from build123d import *

# Parameters (mm, degrees)
SZKIC1_W                                            = 40
SZKIC1_H                                            = 20
POG_BIENIE_WALCOWE_POD_M8_WKR_T_Z_BEM_W_D           = 9
POG_BIENIE_WALCOWE_POD_M8_WKR_T_Z_BEM_W_CBORE_D     = 15
POG_BIENIE_WALCOWE_POD_M8_WKR_T_Z_BEM_W_CBORE_DEPTH = 8.6


with BuildPart() as part:
    # Szkic1 → Obrót1 (revolve)
    with BuildSketch(Plane.XY):
        with Locations((-130, -1.468948521)):
            Rectangle(SZKIC1_W, SZKIC1_H)
    revolve(axis=Axis((0, 8.531051479, 0), (0, -1, 0)))

    # Pogłębienie walcowe pod M8 Wkręt z łbem walcowym z gniazdem sześciokątnym1 (through all)
    with Locations(Plane(origin=(2.665933908, 8.531051479, 0), x_dir=(1, 0, 0), z_dir=(0, 1, 0))):
        with Locations((-139.982449122, 0), (-71.324191515, 118.919590535), (65.9923237, 118.919590535), (134.650581307, 0), (65.9923237, -118.919590535), (-71.324191515, -118.919590535)):
            CounterBoreHole(POG_BIENIE_WALCOWE_POD_M8_WKR_T_Z_BEM_W_D / 2, POG_BIENIE_WALCOWE_POD_M8_WKR_T_Z_BEM_W_CBORE_D / 2, POG_BIENIE_WALCOWE_POD_M8_WKR_T_Z_BEM_W_CBORE_DEPTH)


solid = part.part
Could you check a few things on this model? Use its own coordinates, in mm. A direction names the side the tool comes from. Give positions to 0.01 mm unless a question says otherwise; leave off trailing zeros. Order: outer loops, then holes, each group sorted by start corner. A loop starts at its lowest first (then second) coordinate and runs counter-clockwise, first axis right, second up. Notation, with made-up numbers: (1.5, 3) - (32.5, 3) arc R15 ccw to (32.5, 9) - close; hole circle Ø9 at (14, 38). An arc over 180 degrees is marked (long way). Return JSON: item names as keys, results as strings. Group by question number.
Q1. Suppose I cut it at C-C, the plane y = 3.5. Please give me the cut outline in (x, z).
Q2. Please list where these lines run through material, in increasing order: line 1 along X through (y, z) = (-1.25, -117.5); line 2 along X through (y, z) = (7, 124.5); line 3 along Z through (x, y) = (-71.5, 6.75). Write a range as [from, to].
Q3. Will these pins go through, and if not, where does the flat tip stop? pin 1 Ø8 at (y, z) = (2.5, 25) entering from -X; pin 2 Ø4.5 at (x, z) = (-70, -121.5) entering from +Y; pin 3 Ø1 at (y, z) = (-3, -53) entering from +X.
Q4. Thinking about a two-plate mould opening in Z: for faces 3 (the face through (66.58, -5.85, 122.91)), 4 (the face through (-65, -0.069, 122)), 5 (the face through (67, 8.531, 88)), 6 (the face through (19.527, -1.329, -148.724)), which applies, pulls with the +Z half, pulls with the -Z half, needs draft (parallel to the pull), parting line crosses it, or undercut?
Q5. Suppose I cut it at B-B, the plane z = 0. Please give me the cut outline in (x, y), and give its area (3 significant figures).
Q6. Which directions (+Z, -Z, +X, -X, +Y, -Y) give clear straight access to the entire face, cutting with the end or side of a thin tool? Please do faces 1 (the face through (141, -0.069, 3)), 2 (the face through (133.16, -5.85, 1.72)).
Q7. Suppose I cut it at A-A, the plane x = 0. Please give me the cut outline in (y, z).
Q8. Suppose I cut it at D-D, the plane z = 101. Please give me the cut outline in (x, y), and give its area (3 significant figures).
Resolved:
{
 "1": {"outline": "circle Ø300 at (0, 0); hole circle Ø15 at (-137.32, 0); hole circle Ø220 at (0, 0); hole circle Ø15 at (-68.66, -118.92); hole circle Ø15 at (-68.66, 118.92); hole circle Ø15 at (68.66, -118.92); hole circle Ø15 at (68.66, 118.92); hole circle Ø15 at (137.32, 0)"},
 "2": {"line 1": "x = [-93.24, -72.93], [-64.39, 64.39], [72.93, 93.24]", "line 2": "x = [-83.66, -73.67], [-63.65, 63.65], [73.67, 83.66]", "line 3": "z = [-131.86, -125.86], [-111.98, -83.59], [83.59, 111.98], [125.86, 131.86]"},
 "3": {"pin 1": "stops at x = -148.52", "pin 2": "stops at y = -0.07", "pin 3": "stops at x = 140.51"},
 "4": {"face 3": "undercut", "face 4": "undercut", "face 5": "needs draft", "face 6": "parting line crosses it"},
 "5": {"outline": "(-150, -11.47) - (-141.82, -11.47) - (-141.82, -0.07) - (-144.82, -0.07) - (-144.82, 8.53) - (-150, 8.53) - close; (-132.82, -11.47) - (-110, -11.47) - (-110, 8.53) - (-129.82, 8.53) - (-129.82, -0.07) - (-132.82, -0.07) - close; (110, -11.47) - (132.82, -11.47) - (132.82, -0.07) - (129.82, -0.07) - (129.82, 8.53) - (110, 8.53) - close; (141.82, -11.47) - (150, -11.47) - (150, 8.53) - (144.82, 8.53) - (144.82, -0.07) - (141.82, -0.07) - close", "area": "1,140 mm2"},
 "6": {"face 1": "+Y", "face 2": "+Y, -Y"},
 "7": {"outline": "(-11.47, -150) - (8.53, -150) - (8.53, -110) - (-11.47, -110) - close; (-11.47, 110) - (8.53, 110) - (8.53, 150) - (-11.47, 150) - close"},
 "8": {"outline": "(-110.9, -11.47) - (-43.58, -11.47) - (-43.58, 8.53) - (-110.9, 8.53) - close; (43.58, -11.47) - (110.9, -11.47) - (110.9, 8.53) - (43.58, 8.53) - close", "area": "2,690 mm2"}
}
